Could you check a few things on this model? Use its own coordinates, in mm. Face numbers are marked on the shaded views. A direction names the side the tool comes from. Give positions to 0.01 mm unless a question says otherwise; leave off trailing zeros. Order: outer loops, then holes, each group sorted by start corner. A loop starts at its lowest first (then second) coordinate and runs counter-clockwise, first axis right, second up. Notation, with made-up numbers: (73, 74) -> (108, 74) arc R12 cw to (108, 94) -> close; hole circle Ø8 at (43.5, 36.25). An arc over 180 degrees is marked (long way). Answer as CSV lines item,"result". Start each with the question number.
(1) We'd pull the mould along Z, two halves only. Please class the marked faces 1, 2 and 3: released by +Z, released by -Z, zero draft, split by the parting line, or undercut.
(2) Will these pins go through, and if not, where does the flat tip stop? pin 1 Ø5 at (y, z) = (-2.5, 28.5) entering from -X; pin 2 Ø6 at (y, z) = (-17.68, 42.68) entering from -X; pin 3 Ø7.5 at (x, y) = (3.5, 4) entering from +Z; pin 4 Ø9 at (x, z) = (-14.14, 10.86) entering from +Y.
(3) I need wall thicknesses on L1, parallel to X at y = -15, z = 1; L2, parallel to Z at x = -15, y = 2; L3, parallel to Y at x = -12, z = 1. Which ranges of each line are inside material? Lowest first, please.
(4) On a 3-axis mill with a long thin cutter (end or side, diameter ignored), from which of +Z, -Z, +X, -X, +Y, -Y can I reach the whole of each face in a straight line? I mean the marked faces 4, 5, 6 and 7. Say none if no direction works.
(5) I want a section at B-B (z = 25). Please give me the cut outline in (x, y).
(6) I want a section at A-A (x = 0). Please give me the cut outline in (y, z), plus the area to 3 significant figures.
```python
from build123d import *

# Parameters (mm, degrees)
F0_W      = 50
F0_H      = 50
F1_DEPTH  = 50
F2_R      = 12.5
F3_DEPTH  = 2
F4_R      = 5
F5_DEPTH  = 2
F6_R      = 5
F7_DEPTH  = 2
F8_R      = 5
F9_DEPTH  = 2
F10_R     = 5
F11_DEPTH = 2
F12_R     = 5
F13_DEPTH = 2


with BuildPart() as f1:
    # F0 (on Top) → F1 (new body)
    with BuildSketch(Plane.XY):
        Rectangle(F0_W, F0_H)
    extrude(amount=F1_DEPTH)

    # F2 (on face) → F3 (cut)
    with BuildSketch(Plane.XY.offset(50)):
        Circle(F2_R)
    extrude(amount=-F3_DEPTH, mode=Mode.SUBTRACT)

    # F4 (on face) → F5 (cut)
    with BuildSketch(Plane.YZ.offset(25)):
        with Locations((-10.606602, 35.606602)):
            Circle(F4_R)
        with Locations((10.606602, 14.393398)):
            Circle(F4_R)
    extrude(amount=-F5_DEPTH, mode=Mode.SUBTRACT)

    # F6 (on face) → F7 (cut)
    with BuildSketch(Plane(origin=(0, 25, 0), x_dir=(-1, 0, 0), z_dir=(0, 1, 0))):
        with Locations((0, 25)):
            Circle(F6_R)
        with Locations((-14.142136, 39.142136)):
            Circle(F6_R)
        with Locations((14.142136, 10.857864)):
            Circle(F6_R)
    extrude(amount=-F7_DEPTH, mode=Mode.SUBTRACT)

    # F8 (on face) → F9 (cut)
    with BuildSketch(Plane.XZ.offset(25)):
        with Locations((14.142136, 39.142136)):
            Circle(F8_R)
        with Locations((-14.142136, 39.142136)):
            Circle(F8_R)
        with Locations((-14.142136, 10.857864)):
            Circle(F8_R)
        with Locations((14.142136, 10.857864)):
            Circle(F8_R)
    extrude(amount=-F9_DEPTH, mode=Mode.SUBTRACT)

    # F10 (on face) → F11 (cut)
    with BuildSketch(Plane(origin=(-25, 0, 0), x_dir=(0, -1, 0), z_dir=(-1, 0, 0))):
        with Locations((-17.67767, 42.67767)):
            Circle(F10_R)
        with Locations((0, 25)):
            Circle(F10_R)
        with Locations((-17.67767, 7.32233)):
            Circle(F10_R)
        with Locations((17.67767, 7.32233)):
            Circle(F10_R)
        with Locations((17.67767, 42.67767)):
            Circle(F10_R)
    extrude(amount=-F11_DEPTH, mode=Mode.SUBTRACT)

    # F12 (on face) → F13 (cut)
    with BuildSketch(Plane(origin=(0, 0, 0), x_dir=(1, 0, 0), z_dir=(0, 0, -1))):
        with Locations((-12.5, 15)):
            Circle(F12_R)
        with Locations((-12.5, 0)):
            Circle(F12_R)
        with Locations((-12.5, -15)):
            Circle(F12_R)
        with Locations((12.5, -15)):
            Circle(F12_R)
        with Locations((12.5, 0)):
            Circle(F12_R)
        with Locations((12.5, 15)):
            Circle(F12_R)
    extrude(amount=-F13_DEPTH, mode=Mode.SUBTRACT)


solid = f1.part
```
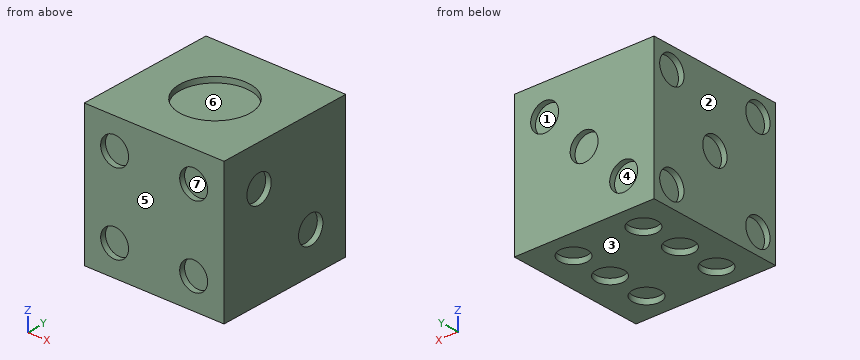
Final values:
1,face 1,"undercut"
1,face 2,"zero draft"
1,face 3,"released by -Z"
2,pin 1,"x = -25"
2,pin 2,"x = -23"
2,pin 3,"z = 48"
2,pin 4,"y = 23"
3,L1,"-25 to -17.5, -7.5 to 7.5, 17.5 to 25"
3,L2,"2 to 50"
3,L3,"-25 to -19.97, -10.03 to -4.97, 4.97 to 10.03, 19.97 to 25"
4,face 4,"+Y"
4,face 5,"+Z, -Z, +X, -X, -Y"
4,face 6,"+Z"
4,face 7,"-Y"
5,outline,"(-25, -25) -> (25, -25) -> (25, 25) -> (5, 25) -> (5, 23) -> (-5, 23) -> (-5, 25) -> (-25, 25) -> (-25, 5) -> (-23, 5) -> (-23, -5) -> (-25, -5) -> close"
6,outline,"(-25, 0) -> (25, 0) -> (25, 20) -> (23, 20) -> (23, 30) -> (25, 30) -> (25, 50) -> (12.5, 50) -> (12.5, 48) -> (-12.5, 48) -> (-12.5, 50) -> (-25, 50) -> close"
6,area,"2,430 mm²"
